Design review of the part built by this model. Coordinates are the model's own, in mm. Face numbers are marked on the shaded views. A direction names the side the tool comes from. Coordinates: 2 decimals unless noted, no trailing zeros. Order: outer loops, then holes, each group sorted by start corner. A loop starts at its lowest first (then second) coordinate and runs counter-clockwise, first axis right, second up. Notation, with made-up numbers: (68.5, 85) -> (83.5, 85) arc R34 cw to (83.5, 118) -> close; hole circle Ø7 at (-3, -38.75). An arc over 180 degrees is marked (long way). Use a Markdown table: item, result. Add a question column.
Q1. Wall thickness on probe 1 along X at (y, z) = (16.5, 0.9); probe 2 along X at (y, z) = (16, 1): over which ranges is each line inside the solid? List them lowest first.
Q2. Add section A-A (z = 35). State the section outline as (x, y) points, then the cut area to 3 significant figures.
Q3. Add section B-B (z = 24.5). State the section outline as (x, y) points, then the cut area to 3 significant figures.
Q4. Insertion check: pin 1 (4 mm diameter, centred on x = -4, y = 1.5, fed in from +Z); pin 2 (7 mm diameter, centred on x = 10, y = -8, fed in from -Z); pin 3 (4 mm diameter, centred on y = -7, z = 7.5, fed in from -X). Each pin has a flat end and moves straight along its axis. Give the tip position at first contact, or say it passes through.
Q5. The part is to be moulded in two halves that separate along Z. For the marked faces 1, 2 and 3, say which applies: pulls with the +Z half, pulls with the -Z half, needs draft (parallel to the pull), parting line crosses it, or undercut.
Q6. Machinability: for the marked faces 4, 5, 6 and 7, which of the approach directions +Z, -Z, +X, -X, +Y, -Y give a long, thin tool a straight path to every point of the face, cutting with its end or side? Answer none if there is none.
from build123d import *

# Parameters (mm, degrees)
F3_DEPTH = 2
F4_R     = 7
F2_R     = 1.1604986379
F5_DEPTH = 2
F6_R     = 1.5
F7_DEPTH = 2


with BuildPart() as f1:
    # F0 (on Front) → F1 (revolve)
    with BuildSketch(Plane.XZ):
        Polygon((-20, 0), (0, 0), (0, 40), (-1.5, 40), (-1.5, 28), (-4.5, 28), (-4.5, 26), (-9.5, 26), (-14, 23), (-14, 5), (-13, 2), (-20, 2), align=None)
    revolve(axis=Axis((0, 0, 20), (0, 0, 1)))

    # F2 (on face) → F3 (cut)
    with BuildSketch(Plane(origin=(0, 0, 0), x_dir=(1, 0, 0), z_dir=(0, 0, -1))):
        with BuildLine():
            Line((-3.75, 3.75), (-3.75, 16.25))
            ThreePointArc((-3.75, 16.25), (-2.6516504294, 18.9016504294), (0, 20))
            ThreePointArc((0, 20), (-14.1421355915, 14.1421356559), (-20, 9.1e-08))
            ThreePointArc((-20, 9.1e-08), (-18.9016503973, 2.6516504616), (-16.25, 3.75))
            Line((-16.25, 3.75), (-3.75, 3.75))
        make_face()
        with BuildLine():
            ThreePointArc((0, 20), (2.6516504294, 18.9016504294), (3.75, 16.25))
            Line((3.75, 16.25), (3.75, 3.75))
            Line((3.75, 3.75), (16.25, 3.75))
            ThreePointArc((16.25, 3.75), (18.9016504294, 2.6516504294), (20, 0))
            ThreePointArc((20, 0), (14.1421356237, 14.1421356237), (0, 20))
        make_face()
        with BuildLine():
            ThreePointArc((-2.95e-08, -20), (14.1421356133, -14.1421356341), (20, 0))
            ThreePointArc((20, 0), (18.9016504294, -2.6516504294), (16.25, -3.75))
            Line((16.25, -3.75), (3.75, -3.75))
            Line((3.75, -3.75), (3.75, -16.25))
            ThreePointArc((3.75, -16.25), (2.651650419, -18.9016504399), (-2.95e-08, -20))
        make_face()
        with BuildLine():
            ThreePointArc((-16.25, -3.75), (-18.9016504616, -2.6516503973), (-20, 9.1e-08))
            ThreePointArc((-20, 9.1e-08), (-14.1421356663, -14.1421355811), (-2.95e-08, -20))
            ThreePointArc((-2.95e-08, -20), (-2.6516504399, -18.901650419), (-3.75, -16.25))
            Line((-3.75, -16.25), (-3.75, -3.75))
            Line((-3.75, -3.75), (-16.25, -3.75))
        make_face()
    extrude(amount=-F3_DEPTH, mode=Mode.SUBTRACT)

    # F4
    f4_edges = [f1.edges().sort_by_distance(p)[0] for p in [
        (3.75, 3.75, 1),
        (-3.75, 3.75, 1),
        (-3.75, -3.75, 1),
        (3.75, -3.75, 1),
    ]]
    fillet(f4_edges, radius=F4_R)

    # F2 (on face) → F5 (cut)
    with BuildSketch(Plane(origin=(0, 0, 0), x_dir=(1, 0, 0), z_dir=(0, 0, -1))):
        Circle(F2_R)
    extrude(amount=-F5_DEPTH, mode=Mode.SUBTRACT)

    # F6 (on face) → F7 (cut)
    with BuildSketch(Plane(origin=(0, 0, 0), x_dir=(1, 0, 0), z_dir=(0, 0, -1))):
        with BuildLine():
            ThreePointArc((1.5, 16.5), (-1.0606601718, 17.5606601718), (0, 15))
            ThreePointArc((0, 15), (1.0606601718, 15.4393398282), (1.5, 16.5))
        make_face()
        with Locations((-16.5, 0)):
            Circle(F6_R)
        with BuildLine():
            ThreePointArc((1.5, -16.5), (1.0606601718, -15.4393398282), (0, -15))
            ThreePointArc((0, -15), (-1.0606601718, -17.5606601718), (1.5, -16.5))
        make_face()
        with BuildLine():
            ThreePointArc((18, 0), (16.5, 1.5), (15, 0))
            ThreePointArc((15, 0), (16.5, -1.5), (18, 0))
        make_face()
    extrude(amount=-F7_DEPTH, mode=Mode.SUBTRACT)


solid = f1.part
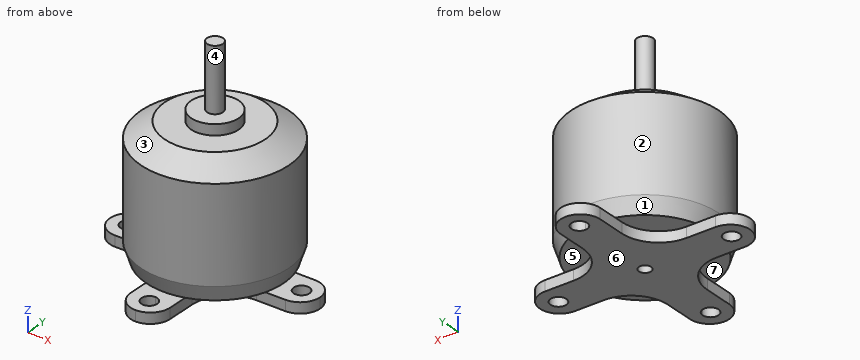
Established:
| question | item | result |
|---|---|---|
| 1 | probe 1 | -3.74 to -1.5, 1.5 to 3.74 |
| 1 | probe 2 | -3.75 to -1.41, 1.41 to 3.75 |
| 2 | outline | circle Ø3 at (0, 0) |
| 2 | area | 7.07 mm^2 |
| 3 | outline | circle Ø23.5 at (0, 0) |
| 3 | area | 434 mm^2 |
| 4 | pin 1 | z = 28 |
| 4 | pin 2 | z = 2 |
| 4 | pin 3 | x = -13.08 |
| 5 | face 1 | undercut |
| 5 | face 2 | needs draft |
| 5 | face 3 | pulls with the +Z half |
| 6 | face 4 | +Z |
| 6 | face 5 | -Z, +X, +Y |
| 6 | face 6 | -Z, +X, -X, +Y, -Y |
| 6 | face 7 | -Z, -X, -Y |
